Design review of the part built by this model. Coordinates are the model's own, in mm. Give positions to 0.01 mm unless a question says otherwise; leave off trailing zeros. Write each loop counter-clockwise with the first axis right and the second up, starting at its lowest first coordinate (ties: lowest second). Pieces come first, ordered by that corner, then holes. Notation, with made-up numbers: M 78,-36 L 123,-36 A24 cw 123,-4 Z; hole C 48.25,-2 d3. An arc over 180 degrees is marked long. Use a Markdown table: item, result. Add a question column.
```python
from build123d import *

# Parameters (mm, degrees)
SKETCH1_R  = 1.016
SKETCH1_W  = 3.175
SKETCH1_H  = 0.2
BASE_DEPTH = 2.7


with BuildPart() as part:
    # Sketch1 → Base (new body)
    with BuildSketch(Plane.XY):
        Polygon((-34.517386137, -9.480737498), (-34.517386137, 13.201100992), (-31.817386137, 13.201100992), (-31.817386137, 23.701100992), (-34.517386137, 23.701100992), (-34.517386137, 33.701100992), (-31.817386137, 33.701100992), (-31.817386137, 52.561262502), (28.182613863, 52.561262502), (28.182613863, 33.701100992), (30.882613863, 33.701100992), (30.882613863, 23.701100992), (28.182613863, 23.701100992), (28.182613863, 13.201100992), (30.882613863, 13.201100992), (30.882613863, -9.480737498), (35.682613863, -9.480737498), (35.682613863, -12.180737498), (43.182613863, -12.180737498), (43.182613863, -9.480737498), (45.482613863, -9.480737498), (45.482613863, 13.121905033), (48.150227726, 13.121905033), (48.150227726, 23.701100992), (45.515, 23.701100992), (45.515, 33.701100992), (48.150227726, 33.701100992), (48.150227726, 72.561262502), (-51.785, 72.561262502), (-51.785, 33.701100992), (-49.149772274, 33.701100992), (-49.149772274, 23.701100992), (-51.785, 23.701100992), (-51.785, 13.121905033), (-49.117386137, 13.121905033), (-49.117386137, -9.480737498), (-46.817386137, -9.480737498), (-46.817386137, -12.180737498), (-39.317386137, -12.180737498), (-39.317386137, -9.480737498), align=None)
        with Locations(Location((-40.7925, 62.561262502, 0), (0, 0, 180))):
            Circle(SKETCH1_R, mode=Mode.SUBTRACT)
        with Locations(Location((38.215, 62.561262502, 0), (0, 0, 180))):
            Circle(SKETCH1_R, mode=Mode.SUBTRACT)
        with Locations(Location((-1.785, 62.561262502, 0), (0, 0, 180))):
            Circle(SKETCH1_R, mode=Mode.SUBTRACT)
        with Locations((-13.247386137, 60.661262502)):
            Rectangle(SKETCH1_W, SKETCH1_H, mode=Mode.SUBTRACT)
        with Locations((-5.627386137, 60.661262502)):
            Rectangle(SKETCH1_W, SKETCH1_H, mode=Mode.SUBTRACT)
        with Locations((1.992613863, 60.661262502)):
            Rectangle(SKETCH1_W, SKETCH1_H, mode=Mode.SUBTRACT)
        with Locations((9.612613863, 60.661262502)):
            Rectangle(SKETCH1_W, SKETCH1_H, mode=Mode.SUBTRACT)
    extrude(amount=BASE_DEPTH)


solid = part.part
```
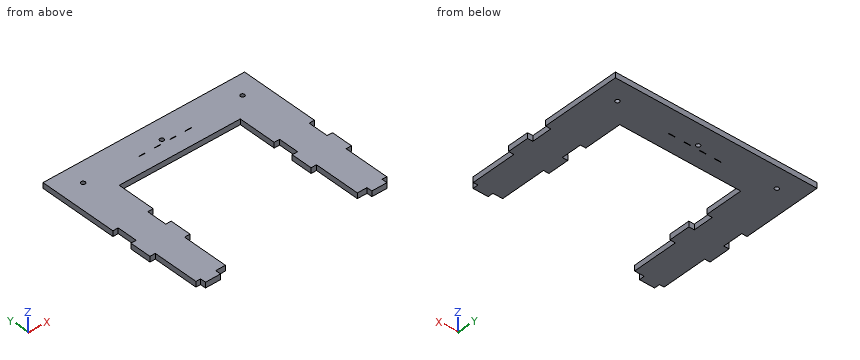
(1) For pin 1 (0.8 mm diameter, centred on y = 6, z = 1, fed in from -X); pin 2 (0.8 mm diameter, centred on x = -50, z = 1, fed in from -Y); pin 3 (1.3 mm diameter, centred on y = -10.5, z = 1.5, fed in from +X), all flat-tipped, find the tip position at first contact; note any pin that passes through.
(2) Add section B-B on y = 45.5. Give the boundary of the cut face in (x, z) (3 decimals).
(3) Add section C-C on x = 22. Give the boundary of the cut face in (y, z), then the cut area to 3 significant figures.
(4) Add section D-D on z = 1. Give the number of separate pieces and of enclosed holes in the cut face, then the cut area to 3 significant figures.
(5) Add section A-A on x = 1.5. Give the boundary of the cut face in (y, z).
(6) Wall thickness on L1, parallel to X at y = 13, z = 1.8; L2, parallel to X at y = 50, z = 1.5 (3 decimals); L3, parallel to Y at x = 1, z = 0.7: over which ranges is each line inside the solid? List them lowest first.
From the geometry:
| question | item | result |
|---|---|---|
| 1 | pin 1 | stops at x = -49.12 |
| 1 | pin 2 | stops at y = 13.12 |
| 1 | pin 3 | stops at x = 43.18 |
| 2 | outline | M -51.785,0 L -31.817,0 L -31.817,2.7 L -51.785,2.7 Z; M 28.183,0 L 48.15,0 L 48.15,2.7 L 28.183,2.7 Z |
| 3 | outline | M 52.56,0 L 72.56,0 L 72.56,2.7 L 52.56,2.7 Z |
| 3 | area | 54.0 mm^2 |
| 4 | separate pieces | 1 |
| 4 | enclosed holes | 7 |
| 4 | area | 4,150 mm^2 |
| 5 | outline | M 52.56,0 L 60.56,0 L 60.56,2.7 L 52.56,2.7 Z; M 60.76,0 L 72.56,0 L 72.56,2.7 L 60.76,2.7 Z |
| 6 | L1 | x = -49.12 to -34.52, 30.88 to 45.48 |
| 6 | L2 | x = -51.785 to -31.817, 28.183 to 48.15 |
| 6 | L3 | y = 52.56 to 60.56, 60.76 to 72.56 |
